```python
from build123d import *

# Parameters (mm, degrees)
F1_DEPTH = 10
F2_R     = 1.689949
F3_R     = 5


with BuildPart() as f1:
    # F0 (on Top) → F1 (new body)
    with BuildSketch(Plane.XY):
        Polygon((0, 10), (0, 0), (18, 0), (18, -16), (13, -16), (0, -13.8), (0, -23.8), (30, -23.8), (30, 10), align=None)
    extrude(amount=F1_DEPTH)

    # F2
    f2_edges = [f1.edges().sort_by_distance(p)[0] for p in [
        (18, 0, 5),
        (18, -16, 5),
        (13, -16, 5),
    ]]
    fillet(f2_edges, radius=F2_R)

    # F3
    f3_edges = [f1.edges().sort_by_distance(p)[0] for p in [
        (0, 10, 5),
        (30, 10, 5),
        (30, -23.8, 5),
        (0, -23.8, 5),
    ]]
    fillet(f3_edges, radius=F3_R)


solid = f1.part
```
Could you check a few things on this model? Use its own coordinates, in mm. A direction names the side the tool comes from. Give positions to 0.01 mm unless a question says otherwise; leave off trailing zeros. Order: outer loops, then holes, each group sorted by start corner. A loop starts at its lowest first (then second) coordinate and runs counter-clockwise, first axis right, second up.
Q1. For faces 1 (the flat face through (15, 10, 5)), 2 (the flat face through (6.5, -14.9, 4.9)), 3 (the flat face through (8, 0, 5)), which set-ups out of +Z, -Z, +X, -X, +Y, -Y let a thin tool reach every point of the face, with its end or its side?
Q2. If I drill on line 1 along Y through (x, z) = (5, 2); line 2 along X through (y, z) = (-7.5, 3.75); line 3 along Y through (x, z) = (9.5, 5.5), over which ranges is the centre line in solid material (lowest first)?
Q3. Suppose I cut it at C-C, the plane x = 11. Write out the boundary of the cut face in (y, z).
Q4. We'd pull the mould along X, two halves only. Please class faces 4 (the cylindrical face through (1, 8, 5)), 5 (the flat face through (15, -16, 5)), 6 (the cylindrical face through (17.52, -15.49, 5.07)), 7 (the flat face through (15, -23.8, 5)): +X half, -X half, draft (parallel to the pull), parting line (faces both ways), or undercut.
Q5. Suppose I cut it at A-A, the plane x = 6.75. Write out the boundary of the cut face in (y, z), and give its area (3 significant figures).
Q6. Suppose I cut it at D-D, the plane y = -5. Write out the boundary of the cut face in (x, z), and give its area (3 significant figures).
Q7. Suppose I cut it at B-B, the plane z = 4.5. Write out the boundary of the cut face in (x, y), and give its area (3 significant figures).
Solution:
1. face 1: +Z, -Z, +X, -X, +Y
1. face 2: +Z, -Z
1. face 3: +Z, -Z, -X
2. line 1: y = -23.8 to -14.65, 0 to 10
2. line 2: x = 18 to 30
2. line 3: y = -23.8 to -15.41, 0 to 10
3. outline: (-23.8, 0) - (-15.66, 0) - (-15.66, 10) - (-23.8, 10) - close; (0, 0) - (10, 0) - (10, 10) - (0, 10) - close
4. face 4: -X half
4. face 5: undercut
4. face 6: undercut
4. face 7: draft
5. outline: (-23.8, 0) - (-14.94, 0) - (-14.94, 10) - (-23.8, 10) - close; (0, 0) - (10, 0) - (10, 10) - (0, 10) - close
5. area: 189 mm2
6. outline: (18, 0) - (30, 0) - (30, 10) - (18, 10) - close
6. area: 120 mm2
7. outline: (0, -18.8) arc R5 ccw to (5, -23.8) - (25, -23.8) arc R5 ccw to (30, -18.8) - (30, 5) arc R5 ccw to (25, 10) - (5, 10) arc R5 ccw to (0, 5) - (0, 0) - (16.31, 0) arc R1.69 cw to (18, -1.69) - (18, -14.31) arc R1.69 cw to (16.31, -16) - (13.14, -16) arc R1.69 cw to (12.86, -15.98) - (0, -13.8) - close
7. area: 720 mm2
